Build history of the part. All positions in model axes, mm. Face numbers are marked on the shaded views. A direction names the side the tool comes from. Round coordinates to 2 decimals unless told otherwise and drop trailing zeros. Loops run counter-clockwise (first coordinate to the right, second up) from the corner with the lowest first, then second, coordinate; pieces in that order, holes last. Notation, with made-up numbers: M -30,69.25 L 20,69.25 A14 cw 20,94.25 Z; hole C -1,38 d4. An arc over 180 degrees is marked long. Use one line per item in the form item = value. Start each with the question number.
```python
from build123d import *

# Parameters (mm, degrees)
SKETCH1_R             = 77.5
BOSS_EXTRUDE1_DEPTH   = 22
SKETCH2_R             = 5
CUT_EXTRUDE1_DEPTH    = 112.787745303
SKETCH3_R             = 10
CUT_EXTRUDE2_DEPTH    = 16.571082
CIRPATTERN1_START     = 5.428917945
CIRPATTERN1_OUTLINE_R = 10
CIRPATTERN1_DEPTH     = 16.571082055


# Read off the part's stored shape, not the designer's step: CirPattern1
with BuildPart() as part:
    # Sketch1 → Boss-Extrude1 (new body)
    with BuildSketch(Plane(origin=(0, 0, 0), x_dir=(1, 0, 0), z_dir=(0, 1, 0))):
        with Locations(Location((0, 0, 0), (0, 0, 270))):
            Circle(SKETCH1_R)
    extrude(amount=BOSS_EXTRUDE1_DEPTH)

    # Sketch2 → Cut-Extrude1 (cut, through all)
    with BuildSketch(Plane(origin=(0, 0, 0), x_dir=(1, 0, 0), z_dir=(0, 1, 0))):
        with Locations(Location((0, 0, 0), (0, 0, 270))):
            Circle(SKETCH2_R)
    extrude(amount=CUT_EXTRUDE1_DEPTH, mode=Mode.SUBTRACT)

    # Sketch3 → Cut-Extrude2 (cut)
    with BuildSketch(Plane(origin=(0, 22, 0), x_dir=(1, 0, 0), z_dir=(0, 1, 0))):
        with Locations(Location((-18.470166118, 0, 0), (0, 0, 270))):
            Circle(SKETCH3_R)
    extrude(amount=-CUT_EXTRUDE2_DEPTH, mode=Mode.SUBTRACT)

    # CirPattern1 outline → CirPattern1 (cut)
    with BuildSketch(Plane(origin=(0, 0, 0), x_dir=(1, 0, 0), z_dir=(0, 1, 0)).offset(CIRPATTERN1_START)):
        with Locations((0, -18.470166118)):
            Circle(CIRPATTERN1_OUTLINE_R)
        with Locations((0, 18.470166118)):
            Circle(CIRPATTERN1_OUTLINE_R)
        with Locations((18.470166118, 0)):
            Circle(CIRPATTERN1_OUTLINE_R)
    extrude(amount=CIRPATTERN1_DEPTH, mode=Mode.SUBTRACT)


solid = part.part
```
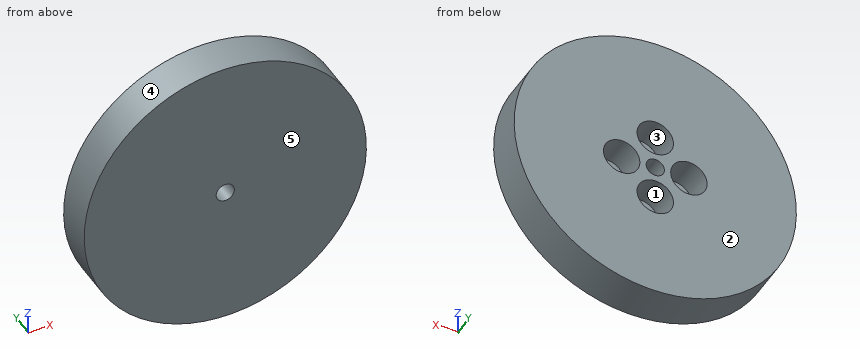
Q1. Saw through at D-D (z = -23.5). Give the cut face in (x, y).
Q2. Saw through at C-C (y = 2.25). Give the cut face in (x, z).
Q3. Saw through at B-B (z = 0). Give the cut face in (x, y).
Q4. Drop flat-ended pins along their axis: P1, Ø6, axis at x = -19, z = 4, coming from the +Y side; P2, Ø6, axis at y = 10.5, z = -45, coming from the -X side; P3, Ø4, axis at x = 33.5, y = 6.5, coming from the +Z side; P4, Ø18, axis at x = 18.47, z = 0, coming from the -Y side. Give the stop position or say it passes through.
Q5. Pull direction X, two halves, no side cores. Call the marked faces 3, 4 and 5: pulls with the +X half, pulls with the -X half, needs draft (parallel to the pull), parting line crosses it, or undercut.
Q6. Wall check: probe 1 along X at (y, z) = (17.5, 0); probe 2 along X at (y, z) = (10, -4); probe 3 along X at (y, z) = (4.25, 0). Give the ranges that are in metal, low to high.
Q7. Tool access for the marked faces 1 and 2: list every direction of +Z, -Z, +X, -X, +Y, -Y with a clear straight run to the whole face (end or side of a thin tool).
Q8. Saw through at A-A (x = 0). Give the cut face in (y, z).
Filled in:
q1.outline = M -73.85,0 L 73.85,0 L 73.85,22 L 8.64,22 L 8.64,5.43 L -8.64,5.43 L -8.64,22 L -73.85,22 Z
q2.outline = C 0,0 d155; hole C 0,0 d10
q3.outline = M -77.5,0 L -5,0 L -5,22 L -8.47,22 L -8.47,5.43 L -28.47,5.43 L -28.47,22 L -77.5,22 Z; M 5,0 L 77.5,0 L 77.5,22 L 28.47,22 L 28.47,5.43 L 8.47,5.43 L 8.47,22 L 5,22 Z
q4.P1 = 5.43
q4.P2 = -65.13
q4.P3 = 70.81
q4.P4 = 0
q5.face_3 = undercut
q5.face_4 = parting line crosses it
q5.face_5 = needs draft
q6.probe_1 = -77.5 to -28.47, -8.47 to -5, 5 to 8.47, 28.47 to 77.5
q6.probe_2 = -77.4 to -27.64, -9.31 to -3, 3 to 9.31, 27.64 to 77.4
q6.probe_3 = -77.5 to -5, 5 to 77.5
q7.face_1 = +Y
q7.face_2 = +Z, -Z, +X, -X, +Y
q8.outline = M 0,-77.5 L 22,-77.5 L 22,-28.47 L 5.43,-28.47 L 5.43,-8.47 L 22,-8.47 L 22,-5 L 0,-5 Z; M 0,5 L 22,5 L 22,8.47 L 5.43,8.47 L 5.43,28.47 L 22,28.47 L 22,77.5 L 0,77.5 Z
